For this review, take the finished solid that the model builds, in its own axes (mm). Give positions to 0.01 mm unless a question says otherwise; leave off trailing zeros. Write each loop counter-clockwise with the first axis right and the second up, starting at its lowest first coordinate (ties: lowest second). Pieces come first, ordered by that corner, then holes. Notation, with made-up numbers: M -4,-27 L 52,-27 A24 ccw 52,-11 Z; hole C -27,56.5 d8. An arc over 180 degrees is marked long. Write item = value, one per line.
```python
from build123d import *

# Parameters (mm, degrees)
SKETCH1_W                   = 88.9
SKETCH1_H                   = 60.325
SOLARPANELPLASTICBASE_DEPTH = 2.54
CRYSTALELEMENT_DEPTH        = 0.5969
OUTSIDEFILLET_R             = 0.8255
LPATTERN1_COUNT             = 5
LPATTERN1_PITCH             = 17.4498
LPATTERN1_COUNT_DIR2        = 2
LPATTERN1_PITCH_DIR2        = 30.48


with BuildPart() as part:
    # Sketch1 → SolarPanelPlasticBase (new body)
    with BuildSketch(Plane.XY):
        Rectangle(SKETCH1_W, SKETCH1_H)
    extrude(amount=SOLARPANELPLASTICBASE_DEPTH)

    # Sketch2 → CrystalElement (add)
    with BuildSketch(Plane.XY.offset(2.54)):
        Polygon((-39.6875, 28.575), (-30.1625, 28.575), (-26.9875, 25.4), (-26.9875, 4.7625), (-30.1625, 1.5875), (-39.6875, 1.5875), (-42.8625, 4.7625), (-42.8625, 25.4), align=None)
    crystalelement = extrude(amount=CRYSTALELEMENT_DEPTH)

    # OutsideFillet
    outsidefillet_edges = [part.edges().sort_by_distance(p)[0] for p in [
        (44.45, 0, 2.54),
        (0, 30.1625, 2.54),
        (-44.45, 0, 2.54),
        (0, -30.1625, 2.54),
    ]]
    fillet(outsidefillet_edges, radius=OUTSIDEFILLET_R)

    # LPattern1: CrystalElement 5 × 2
    with Locations(*[(i * LPATTERN1_PITCH, -j * LPATTERN1_PITCH_DIR2, 0) for i in range(LPATTERN1_COUNT) for j in range(LPATTERN1_COUNT_DIR2) if (i, j) != (0, 0)]):
        add(crystalelement)


solid = part.part
```
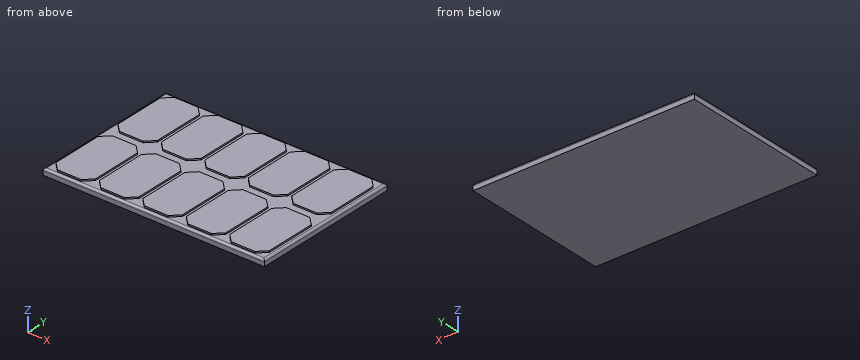
1. We need section A-A, the plane y = -12. Write out the cut boundary in (x, z), then the cut area to 3 significant figures.
Responses:
outline = M -44.45,0 L 44.45,0 L 44.45,1.71 A0.83 ccw 43.62,2.54 L 42.81,2.54 L 42.81,3.14 L 26.94,3.14 L 26.94,2.54 L 25.36,2.54 L 25.36,3.14 L 9.49,3.14 L 9.49,2.54 L 7.91,2.54 L 7.91,3.14 L -7.96,3.14 L -7.96,2.54 L -9.54,2.54 L -9.54,3.14 L -25.41,3.14 L -25.41,2.54 L -26.99,2.54 L -26.99,3.14 L -42.86,3.14 L -42.86,2.54 L -43.62,2.54 A0.83 ccw -44.45,1.71 Z
area = 273 mm2
2. We need section B-B, the plane x = -16. Write out the cut boundary in (y, z) (1 decimal), then the cut area to 3 significant figures.
Responses:
outline = M -30.2,0 L 30.2,0 L 30.2,1.7 A0.8 ccw 29.3,2.5 L 28.6,2.5 L 28.6,3.1 L 1.6,3.1 L 1.6,2.5 L -1.9,2.5 L -1.9,3.1 L -28.9,3.1 L -28.9,2.5 L -29.3,2.5 A0.8 ccw -30.2,1.7 Z
area = 185 mm2
3. For line 1 along X through (y, z) = (-6, 2.6); line 2 along Y through (x, z) = (-39.5, 1.9); line 3 along Z through (x, y) = (-8.5, -16), list the stretches that pass through material, from the lowest coordinate up. Write a range as from..to.
Responses:
line_1 = -42.86..-26.99, -25.41..-9.54, -7.96..7.91, 9.49..25.36, 26.94..42.81
line_2 = -30.14..30.14
line_3 = 0..2.54
4. Insertion check: P1, Ø0.5, axis at x = 36, z = 3, coming from the +Y side (3 decimals); P2, Ø10, axis at x = -20.5, y = 12.5, coming from the -Z side; P3, Ø0.5, axis at y = -17, z = 2.5, coming from the +X side; P4, Ø0.5, axis at y = 19, z = 3, coming from the +X side. Each pin has a flat end and moves straight along its axis. Give the tip position at first contact, or say it passes through.
Responses:
P1 = 28.575
P2 = 0
P3 = 44.25
P4 = 42.81
5. We need section C-C, the plane y = -0.5. Write out the cut boundary in (x, z), then the cut area to 3 significant figures.
Responses:
outline = M -44.45,0 L 44.45,0 L 44.45,1.71 A0.83 ccw 43.62,2.54 L -43.62,2.54 A0.83 ccw -44.45,1.71 Z
area = 226 mm2
